Geometry: final body of the model. Coordinates: model frame, mm. A direction names the side the tool comes from. Round coordinates to 2 decimals unless told otherwise and drop trailing zeros. Write each loop counter-clockwise with the first axis right and the second up, starting at its lowest first coordinate (ties: lowest second). Pieces come first, ordered by that corner, then holes. Notation, with made-up numbers: (8, 82) -> (66, 82) arc R22 cw to (66, 94) -> close; hole circle Ø4 at (22, 41.25). An arc over 180 degrees is marked (long way). Use one line per item in the form item = value. Start each with the question number.
1. Reachability of faces 5 (the face through (6.43, -3.07, 0.4)), 6 (the face through (11.316, -3.036, 2.826)), 7 (the face through (3.568, -0.5, -0.5)) from +Z, -Z, +X, -X, +Y, -Y: full face, straight path, thin tool, end or side. Return the list, or none.
2. Cut plane B-B, the plane x = 8.5. Return the cut outline in (y, z) (1 decimal).
3. Draft query along Y for faces 1 (the face through (12.335, -0.1, -2.4)), 2 (the face through (11.4, 1.91, -0.99)), 3 (the face through (11.316, 3.036, -2.826)), 4 (the face through (3.05, 0.466, -0.242)). Return one class per face: pulls with the +Y half, pulls with the -Y half, needs draft (parallel to the pull), parting line crosses it, or undercut.
4. Line query: L1, parallel to Y at x = 3.3, z = 0 (1 decimal); L2, parallel to X at y = -1, z = 0.25. Output: solid intervals per line, ascending.
5. Pin query (flat end, axial travel): pin 1 Ø4 at (x, y) = (4.5, 1.5) entering from +Z; pin 2 Ø0.6 at (y, z) = (0, 0) entering from +X; pin 3 Ø2 at (x, y) = (4, 3) entering from -Z; pin 4 Ø2 at (x, z) = (10.5, 2) entering from -Y. Return the tip coordinate at first contact, or that it passes through.
```python
from build123d import *

# Parameters (mm, degrees)
ESQUISSE2_OUTSIDE_W                   = 16.214
ESQUISSE2_OUTSIDE_H                   = 16.214
ENL_V_MAT_EXTRU_1_DEPTH               = 17.967468874
ENL_VEMENT_DE_MATI_RE_BALAYAGE2_PITCH = 5.1
R_P_TITION_CIRCULAIRE1_COUNT          = 2
ENL_VEMENT_DE_MATI_RE_BALAYAGE3_PITCH = 0.85
CONG_1_R                              = 0.2
SCALE1_SCALE                          = 1.05


with BuildPart() as part:
    # Esquisse1 → Révolution1 (revolve)
    with BuildSketch(Plane.XY, mode=Mode.PRIVATE) as r_volution1_sk:
        Polygon((10.309090909, 2.95), (5.709090909, 2.95), (5.709090909, 4.55), (3.309090909, 4.55), (2.309090909, 3.175), (-3.190909091, 3.175), (-3.190909091, 1.4), (-4.490909091, 1.075), (-5.690909091, 1.075), (-5.690909091, 1.3), (-8.690909091, 0.85), (-9.990909091, 0.85), (-9.990909091, 0.5), (3.759090909, 0.5), (3.759090909, 1.920326087), (5.709090909, 1.95), (10.309090909, 2.02), (12.109090909, 2.075), (12.109090909, 3.95), (10.309090909, 3.95), align=None)
    revolve(r_volution1_sk.sketch.rotate(Axis((13.255472394, 0, 0), (-1, 0, 0)), 90), axis=Axis((13.255472394, 0, 0), (-1, 0, 0)))

    # Esquisse2 outside → Enlèv. mat.-Extru.1 (cut, through all)
    with BuildSketch(Plane(origin=(5.709090909, 0, 0), x_dir=(0, 0, -1), z_dir=(1, 0, 0))):
        Rectangle(ESQUISSE2_OUTSIDE_W, ESQUISSE2_OUTSIDE_H)
        Polygon((0, -4.618802154), (4, -2.309401077), (4, 2.309401077), (0, 4.618802154), (-4, 2.309401077), (-4, -2.309401077), align=None, mode=Mode.SUBTRACT)
    extrude(amount=-ENL_V_MAT_EXTRU_1_DEPTH, mode=Mode.SUBTRACT)

    # Enlèvement de matière-Balayage2: the profile of Esquisse5 screwed along a right-hand helix of 1.2 turns, 12 arcs to a turn; built about Z, then put on its axis
    enl_vement_de_mati_re_balayage2_z = Axis((0, 0, 0), (0, 0, 1))
    enl_vement_de_mati_re_balayage2_corners = [(4.45, 0, 0), (3.3, 0, -0.66395281), (3.3, 0, -1.86395281), (4.45, 0, -2.527905619)]
    with BuildLine(mode=Mode.PRIVATE) as enl_vement_de_mati_re_balayage2_profile:
        Line(enl_vement_de_mati_re_balayage2_corners[0], enl_vement_de_mati_re_balayage2_corners[1])
        Line(enl_vement_de_mati_re_balayage2_corners[1], enl_vement_de_mati_re_balayage2_corners[2])
        Line(enl_vement_de_mati_re_balayage2_corners[2], enl_vement_de_mati_re_balayage2_corners[3])
        Line(enl_vement_de_mati_re_balayage2_corners[3], enl_vement_de_mati_re_balayage2_corners[0])
    enl_vement_de_mati_re_balayage2_cap = Face(enl_vement_de_mati_re_balayage2_profile.wire())
    enl_vement_de_mati_re_balayage2_turn_angles = [0, 15, 30, 45, 60, 75, 90, 105, 120, 135, 150, 165, 180, 195, 210, 225, 240, 255, 270, 285, 300, 315, 330, 345, 360]
    enl_vement_de_mati_re_balayage2_turn_weights = [1, 0.9659258262890683, 1, 0.9659258262890683, 1, 0.9659258262890683, 1, 0.9659258262890683, 1, 0.9659258262890683, 1, 0.9659258262890683, 1, 0.9659258262890683, 1, 0.9659258262890683, 1, 0.9659258262890683, 1, 0.9659258262890683, 1, 0.9659258262890683, 1, 0.9659258262890683, 1]
    enl_vement_de_mati_re_balayage2_turn_rails = [Edge.make_bspline([Vector(p[0], p[1], 0).rotate(enl_vement_de_mati_re_balayage2_z, enl_vement_de_mati_re_balayage2_turn_angles[k]) / enl_vement_de_mati_re_balayage2_turn_weights[k] + Vector(0, 0, p[2] + ENL_VEMENT_DE_MATI_RE_BALAYAGE2_PITCH * enl_vement_de_mati_re_balayage2_turn_angles[k] / 360) for k in range(25)], [0, 0, 0, 1, 1, 2, 2, 3, 3, 4, 4, 5, 5, 6, 6, 7, 7, 8, 8, 9, 9, 10, 10, 11, 11, 12, 12, 12], 2, enl_vement_de_mati_re_balayage2_turn_weights) for p in enl_vement_de_mati_re_balayage2_corners]
    enl_vement_de_mati_re_balayage2_turn_sides = [Face.make_surface_from_curves(enl_vement_de_mati_re_balayage2_turn_rails[p[0]], enl_vement_de_mati_re_balayage2_turn_rails[p[1]]) for p in [(0, 1), (1, 2), (2, 3), (3, 0)]]
    enl_vement_de_mati_re_balayage2_last_angles = [360, 375, 390, 405, 420, 426, 432]
    enl_vement_de_mati_re_balayage2_last_weights = [1, 0.9659258262890683, 1, 0.9659258262890683, 1, 0.9945218953682725, 1]
    enl_vement_de_mati_re_balayage2_last_rails = [Edge.make_bspline([Vector(p[0], p[1], 0).rotate(enl_vement_de_mati_re_balayage2_z, enl_vement_de_mati_re_balayage2_last_angles[k]) / enl_vement_de_mati_re_balayage2_last_weights[k] + Vector(0, 0, p[2] + ENL_VEMENT_DE_MATI_RE_BALAYAGE2_PITCH * enl_vement_de_mati_re_balayage2_last_angles[k] / 360) for k in range(7)], [0, 0, 0, 1, 1, 2, 2, 3, 3, 3], 2, enl_vement_de_mati_re_balayage2_last_weights) for p in enl_vement_de_mati_re_balayage2_corners]
    enl_vement_de_mati_re_balayage2_last_sides = [Face.make_surface_from_curves(enl_vement_de_mati_re_balayage2_last_rails[p[0]], enl_vement_de_mati_re_balayage2_last_rails[p[1]]) for p in [(0, 1), (1, 2), (2, 3), (3, 0)]]
    enl_vement_de_mati_re_balayage2 = Plane(origin=(13.109090909, 0, 0), x_dir=(0, 0, -1), z_dir=(-1, 0, 0)) * Solid(Shell([*enl_vement_de_mati_re_balayage2_turn_sides, *enl_vement_de_mati_re_balayage2_last_sides, enl_vement_de_mati_re_balayage2_cap, enl_vement_de_mati_re_balayage2_cap.rotate(enl_vement_de_mati_re_balayage2_z, 432).moved(Location((0, 0, ENL_VEMENT_DE_MATI_RE_BALAYAGE2_PITCH * 432 / 360)))]))
    add(enl_vement_de_mati_re_balayage2, mode=Mode.SUBTRACT)

    # Répétition circulaire1: Enlèvement de matière-Balayage2 ×2 about axis
    r_p_tition_circulaire1_axis = Axis((3.759090909, 0, 0), (1, 0, 0))
    for i in range(1, R_P_TITION_CIRCULAIRE1_COUNT):
        add(enl_vement_de_mati_re_balayage2.rotate(r_p_tition_circulaire1_axis, i * 360 / R_P_TITION_CIRCULAIRE1_COUNT), mode=Mode.SUBTRACT)

    # Esquisse6 → Enlèvement de matière-Révolution2 (revolve, cut)
    with BuildSketch(Plane(origin=(0, 0, 0), x_dir=(1, 0, 0), z_dir=(0, 0, -1)), mode=Mode.PRIVATE) as enl_vement_de_mati_re_r_volution2_sk:
        with BuildLine():
            Line((5.209090909, 4.598364037), (5.709090909, 4.598364037))
            Line((5.709090909, 4.598364037), (5.709090909, 2.95))
            ThreePointArc((5.709090909, 2.95), (5.581340735, 3.811264187), (5.209090909, 4.598364037))
        make_face()
        Polygon((2.309090909, -3.175), (-3.190909091, -2.95), (-3.190909091, -3.175), align=None)
    revolve(enl_vement_de_mati_re_r_volution2_sk.sketch.rotate(Axis((-1.819283659, 0, 0), (1, 0, 0)), 270), axis=Axis((-1.819283659, 0, 0), (1, 0, 0)), mode=Mode.SUBTRACT)


with BuildPart() as body_2:
    # Fractionner1: the piece on the far side of the plane
    add(part.part)
    split(bisect_by=Plane(origin=(2.309090909, 0, 0), x_dir=(0, 0, 1), z_dir=(1, 0, 0)), keep=Keep.BOTTOM)

    # Enlèvement de matière-Balayage3: the profile of Esquisse8 screwed along a right-hand helix of 12 turns, 8 arcs to a turn; built about Z, then put on its axis
    enl_vement_de_mati_re_balayage3_z = Axis((0, 0, 0), (0, 0, 1))
    enl_vement_de_mati_re_balayage3_corners = [(2.65, 0, -0.05), (2.65, 0, 0.05), (3.3433932, 0, 0.5), (3.3433932, 0, -0.5)]
    with BuildLine(mode=Mode.PRIVATE) as enl_vement_de_mati_re_balayage3_profile:
        Line(enl_vement_de_mati_re_balayage3_corners[0], enl_vement_de_mati_re_balayage3_corners[1])
        Line(enl_vement_de_mati_re_balayage3_corners[1], enl_vement_de_mati_re_balayage3_corners[2])
        Line(enl_vement_de_mati_re_balayage3_corners[2], enl_vement_de_mati_re_balayage3_corners[3])
        Line(enl_vement_de_mati_re_balayage3_corners[3], enl_vement_de_mati_re_balayage3_corners[0])
    enl_vement_de_mati_re_balayage3_cap = Face(enl_vement_de_mati_re_balayage3_profile.wire())
    enl_vement_de_mati_re_balayage3_turn_angles = [0, 22.5, 45, 67.5, 90, 112.5, 135, 157.5, 180, 202.5, 225, 247.5, 270, 292.5, 315, 337.5, 360]
    enl_vement_de_mati_re_balayage3_turn_weights = [1, 0.9238795325112867, 1, 0.9238795325112867, 1, 0.9238795325112867, 1, 0.9238795325112867, 1, 0.9238795325112867, 1, 0.9238795325112867, 1, 0.9238795325112867, 1, 0.9238795325112867, 1]
    enl_vement_de_mati_re_balayage3_turn_rails = [Edge.make_bspline([Vector(p[0], p[1], 0).rotate(enl_vement_de_mati_re_balayage3_z, enl_vement_de_mati_re_balayage3_turn_angles[k]) / enl_vement_de_mati_re_balayage3_turn_weights[k] + Vector(0, 0, p[2] + ENL_VEMENT_DE_MATI_RE_BALAYAGE3_PITCH * enl_vement_de_mati_re_balayage3_turn_angles[k] / 360) for k in range(17)], [0, 0, 0, 1, 1, 2, 2, 3, 3, 4, 4, 5, 5, 6, 6, 7, 7, 8, 8, 8], 2, enl_vement_de_mati_re_balayage3_turn_weights) for p in enl_vement_de_mati_re_balayage3_corners]
    enl_vement_de_mati_re_balayage3_turn_sides = [Face.make_surface_from_curves(enl_vement_de_mati_re_balayage3_turn_rails[p[0]], enl_vement_de_mati_re_balayage3_turn_rails[p[1]]) for p in [(0, 1), (1, 2), (2, 3), (3, 0)]]
    enl_vement_de_mati_re_balayage3 = Plane(origin=(-4.190909091, 0, 0), x_dir=(0, 0, 1), z_dir=(1, 0, 0)) * Solid(Shell([*[p.moved(Location((0, 0, ENL_VEMENT_DE_MATI_RE_BALAYAGE3_PITCH * i))) for i in range(12) for p in enl_vement_de_mati_re_balayage3_turn_sides], enl_vement_de_mati_re_balayage3_cap, enl_vement_de_mati_re_balayage3_cap.rotate(enl_vement_de_mati_re_balayage3_z, 4320).moved(Location((0, 0, ENL_VEMENT_DE_MATI_RE_BALAYAGE3_PITCH * 4320 / 360)))]))
    add(enl_vement_de_mati_re_balayage3, mode=Mode.SUBTRACT)


with BuildPart() as part_1:
    add(part.part)

    # Fractionner1
    split(bisect_by=Plane(origin=(2.309090909, 0, 0), x_dir=(0, 0, 1), z_dir=(1, 0, 0)), keep=Keep.TOP)


with BuildPart() as body_2_1:
    add(body_2.part)

    # Combiner1: union part
    add(part_1.part)

    # Congé1
    cong_1_edges = [body_2_1.edges().sort_by_distance(p)[0] for p in [
        (5.709090909, -2.95, 0),
        (-3.190909091, 0, 1.4),
    ]]
    fillet(cong_1_edges, radius=CONG_1_R)

    # Sketch1 → Cut-Revolve1 (revolve, cut)
    with BuildSketch(Plane(origin=(0, 0, 0), x_dir=(1, 0, 0), z_dir=(0, 1, 0))):
        Polygon((2.759090909, 2.95), (10.307039448, 2.95), (10.307039448, 5.53408659), (-10.725109123, 5.53408659), (-10.725109123, 0.335117348), (2.759090909, 0.335117348), align=None)
        Polygon((10.307039448, -6.163499881), (10.307039448, -2.95), (2.759090909, -2.95), (2.759090909, 0), (-10.725109123, 0), (-10.725109123, -6.163499881), align=None)
    revolve(axis=Axis((-11.213736174, 0, 0), (1, 0, 0)), mode=Mode.SUBTRACT)


with BuildPart() as body_2_2:
    # Scale1: scaled about (7.582829496, 8.827e-06, -7.484e-06)
    add(body_2_1.part.scale(SCALE1_SCALE).moved(Location((-0.379141475, -4.41e-07, 3.74e-07))))


solid = body_2_2.part
```
Outcome:
q1.face_5 = -X
q1.face_6 = +X, -X
q1.face_7 = +X
q2.outline = circle Ø6.2 at (0, 0); hole circle Ø4.2 at (0, 0)
q3.face_1 = needs draft
q3.face_2 = undercut
q3.face_3 = parting line crosses it
q3.face_4 = undercut
q4.L1 = -3.1 to -0.5, 0.5 to 3.1
q4.L2 = 2.52 to 3.57
q5.pin_1 = 3.1
q5.pin_2 = through
q5.pin_3 = -2.37
q5.pin_4 = -3.85
